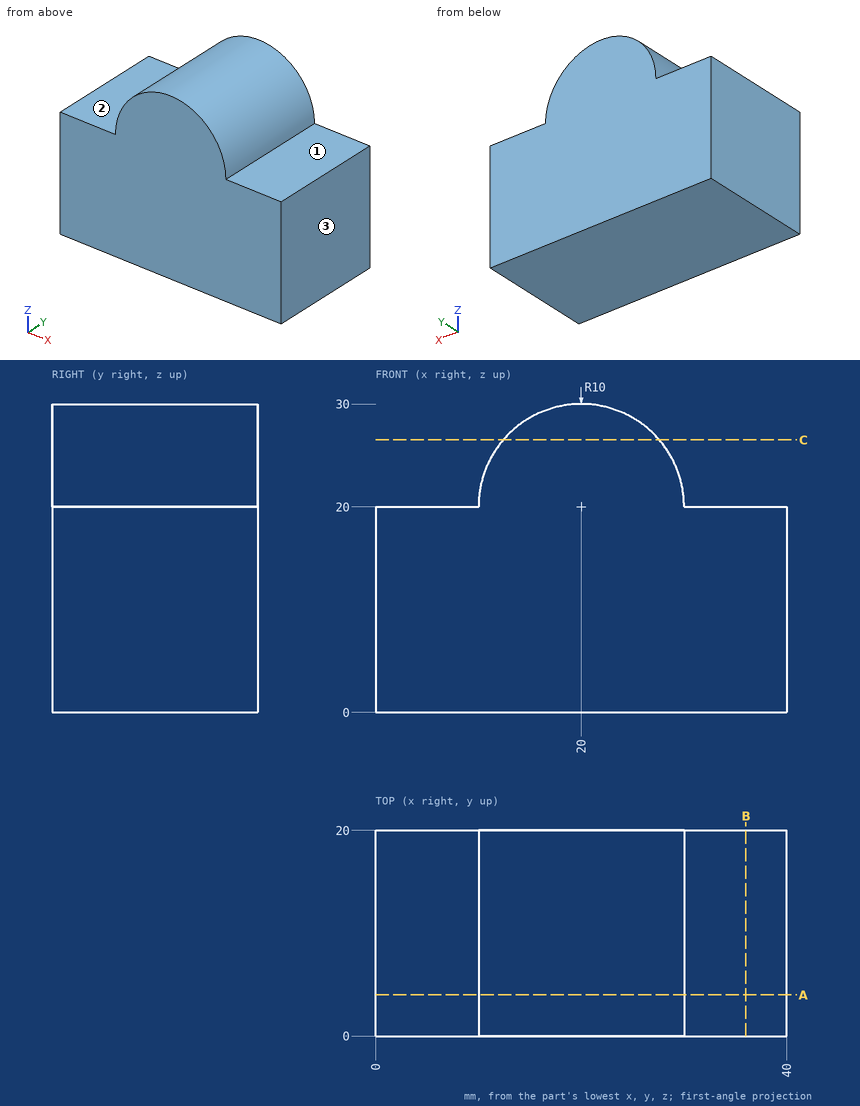
Part print with two shaded views. Sizes in mm from the minimum x, y, z corner. A direction names the side the tool comes from. Round coordinates to 2 decimals unless told otherwise and drop trailing zeros. Order: outer loops, then holes, each group sorted by start corner. A loop starts at its lowest first (then second) coordinate and runs counter-clockwise, first axis right, second up.
(1) Band-saw the part on A-A (y = 4). List the corners of the cut face in (x, z), then the cut area to 3 significant figures.
(2) 3-axis set-ups, long thin cutter, end or side, ignore diameter. For the marked faces 1, 2 and 3: which of +Z, -Z, +X, -X, +Y, -Y reach the whole face in a straight line?
(3) Band-saw the part on C-C (z = 26.5). List the corners of the cut face in (x, y).
(4) Drill centre lines: line 1 (Z direction, x = 35, y = 7.75); line 2 (Z direction, x = 20, y = 9.75); line 3 (X direction, y = 5.25, z = 24.75). Where is each one in solid material? Low to high.
(5) Pin check, flat tips, straight feed: pin 1 (1.5 mm diameter, centred on y = 13, z = 22.5, fed in from +X); pin 2 (1 mm diameter, centred on y = 5, z = 12.5, fed in from -X); pin 3 (12 mm diameter, centred on x = 29.5, y = 10, fed in from +Z); pin 4 (3 mm diameter, centred on y = 4, z = 25.5, fed in from +X). Stop position of each tip, or through.
(6) Band-saw the part on B-B (x = 36). List the corners of the cut face in (y, z), then the cut area to 3 significant figures.
Verdict:
1. outline: (0, 0) - (40, 0) - (40, 20) - (30, 20) arc R10 ccw to (10, 20) - (0, 20) - close
1. area: 957 mm2
2. face 1: +Z, +X, +Y, -Y
2. face 2: +Z, -X, +Y, -Y
2. face 3: +Z, -Z, +X, +Y, -Y
3. outline: (12.4, 0) - (27.6, 0) - (27.6, 20) - (12.4, 20) - close
4. line 1: z = 0 to 20
4. line 2: z = 0 to 30
4. line 3: x = 11.2 to 28.8
5. pin 1: stops at x = 29.85
5. pin 2: stops at x = 0
5. pin 3: stops at z = 29.37
5. pin 4: stops at x = 29.17
6. outline: (0, 0) - (20, 0) - (20, 20) - (0, 20) - close
6. area: 400 mm2
